Here's how the part is built. I have some questions about the finished solid (model axes, mm). Face numbers are marked on the shaded views. A direction names the side the tool comes from. Round coordinates to 2 decimals unless told otherwise and drop trailing zeros. Order: outer loops, then holes, each group sorted by start corner. A loop starts at its lowest first (then second) coordinate and runs counter-clockwise, first axis right, second up. Notation, with made-up numbers: M 12,10 L 23,10 A23 cw 23,32 Z; hole C 3,-28.5 d10. An arc over 180 degrees is marked long. Write item = value, one per line. Start each with the question number.
Item 1: For the marked faces 4 and 5, which set-ups out of +Z, -Z, +X, -X, +Y, -Y let a thin tool reach every point of the face, with its end or its side?
Item 2: Please list where these lines run through material, in increasing order: L1, parallel to Y at x = 0, z = -16; L2, parallel to Z at x = 34.5, y = -10; L3, parallel to X at y = 0, z = -13.
Item 3: I want a section at C-C, the plane z = -8.5. List the corners of the cut face in (x, y) for me.
Item 4: We'd pull the mould along X, two halves only. Please class the marked faces 1, 2 and 3: pulls with the +X half, pulls with the -X half, needs draft (parallel to the pull), parting line crosses it, or undercut.
Item 5: I want a section at B-B, the plane x = 0. List the corners of the cut face in (y, z) for me.
Item 6: I want a section at D-D, the plane z = -37. List the corners of the cut face in (x, y) for me.
Item 7: I want a section at A-A, the plane y = 0. List the corners of the cut face in (x, z) for me, plus the area to 3 significant figures.
Item 8: I'm going to push flat-ended pins straight in: P1, Ø1, axis at x = -55, y = 45.5, coming from the +Z side; P2, Ø2, axis at y = 0, z = -6.5, coming from the -X side; P3, Ø24, axis at x = 6, y = 29, coming from the +Z side; P4, Ø2, axis at x = -7.5, z = -7.5, coming from the +Y side. Where does each tip first touch, or does it pass through?
```python
from build123d import *

# Parameters (mm, degrees)
F1_DEPTH = 40
F3_DEPTH = 35


with BuildPart() as f1:
    # F0 (on Top) → F1 (new body)
    with BuildSketch(Plane.XY):
        with BuildLine():
            Line((-67.082039, -20), (67.082039, -20))
            ThreePointArc((67.082039, -20), (0, 70), (-67.082039, -20))
        make_face()
    extrude(amount=-F1_DEPTH)

    # F2 (on face) → F3 (cut)
    with BuildSketch(Plane.XY):
        with BuildLine():
            Line((-63.245553, -15), (63.245553, -15))
            ThreePointArc((63.245553, -15), (0, 65), (-63.245553, -15))
        make_face()
    extrude(amount=-F3_DEPTH, mode=Mode.SUBTRACT)


solid = f1.part
```
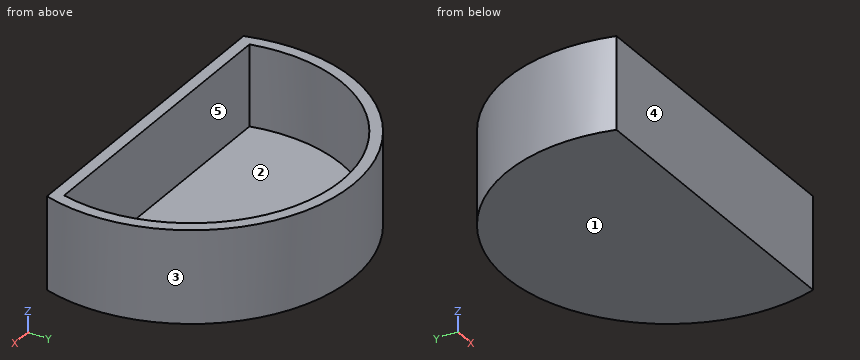
Filled in:
q1.face_4 = +Z, -Z, +X, -X, -Y
q1.face_5 = +Z
q2.L1 = -20 to -15, 65 to 70
q2.L2 = -40 to -35
q2.L3 = -70 to -65, 65 to 70
q3.outline = M -67.08,-20 L 67.08,-20 A70 ccw long Z; hole M -63.25,-15 L 63.25,-15 A65 ccw long Z
q4.face_1 = needs draft
q4.face_2 = undercut
q4.face_3 = parting line crosses it
q5.outline = M -20,-40 L 70,-40 L 70,0 L 65,0 L 65,-35 L -15,-35 L -15,0 L -20,0 Z
q6.outline = M -67.08,-20 L 67.08,-20 A70 ccw long Z
q7.outline = M -70,-40 L 70,-40 L 70,0 L 65,0 L 65,-35 L -65,-35 L -65,0 L -70,0 Z
q7.area = 1,050 mm^2
q8.P1 = through
q8.P2 = -70
q8.P3 = -35
q8.P4 = 69.7
